Geometry check sheet. Reference: drawing and pictorial views, mm from the part's lowest x, y, z. A direction names the side the tool comes from. Coordinates: 2 decimals unless noted, no trailing zeros. Write each loop counter-clockwise with the first axis right and the second up, starting at its lowest first coordinate (ties: lowest second). Pieces come first, ordered by that corner, then holes.
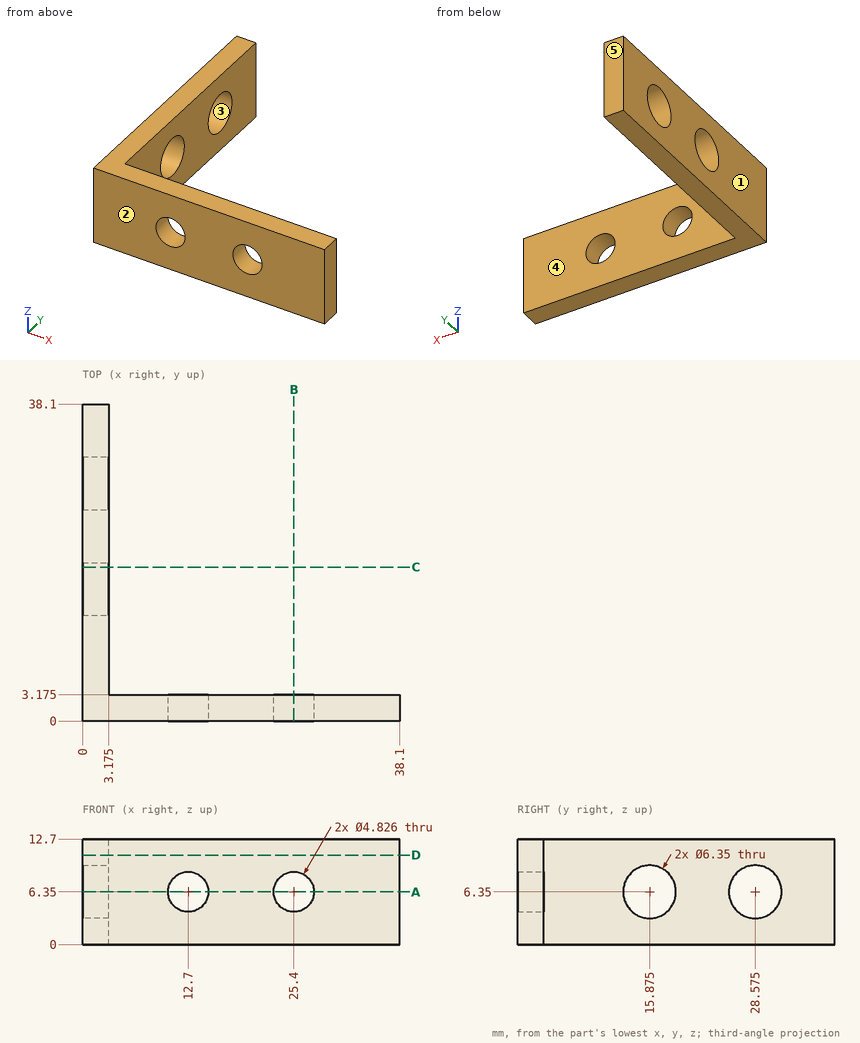
1. Sectioned sample at B-B, the plane x = 25.4. Record the boundary of the cut face in (y, z) (3 decimals).
2. Sectioned sample at D-D, the plane z = 10.75. Record the boundary of the cut face in (x, y) (3 decimals).
3. Material ranges on L1, parallel to X at y = 1.7, z = 6.35; L2, parallel to Y at x = 0.8, z = 6.35; L3, parallel to Y at x = 2, z = 4.25, recorded low to high.
4. Sectioned sample at C-C, the plane y = 18.5. Record the boundary of the cut face in (x, z) (3 decimals), and give its area (3 significant figures).
5. Draft check along Y on the marked faces 1, 2 and 3. Enter one of: pulls with the +Y half, pulls with the -Y half, needs draft (parallel to the pull), parting line crosses it, or undercut.
6. Gauge pin test, flat end, axial feed: P1, Ø1.5, axis at y = 20.5, z = 10, coming from the +X side (3 decimals). Record the tip position at first contact, or that the pin passes through.
7. Sectioned sample at A-A, the plane z = 6.35. Record the boundary of the cut face in (x, y) (3 decimals).
8. Tool access check on the marked faces 4 and 5. Record the directions out of +Z, -Z, +X, -X, +Y, -Y that give a thin tool (end or side, any length) a straight path to the whole face; none if there is none.
Outcome:
1. outline: (0, 0) - (3.175, 0) - (3.175, 3.937) - (0, 3.937) - close; (0, 8.763) - (3.175, 8.763) - (3.175, 12.7) - (0, 12.7) - close
2. outline: (0, 0) - (38.1, 0) - (38.1, 3.175) - (3.175, 3.175) - (3.175, 38.1) - (0, 38.1) - close
3. L1: x = 0 to 10.29, 15.11 to 22.99, 27.81 to 38.1
3. L2: y = 0 to 12.7, 19.05 to 25.4, 31.75 to 38.1
3. L3: y = 0 to 13.49, 18.26 to 26.19, 30.96 to 38.1
4. outline: (0, 0) - (3.175, 0) - (3.175, 4.564) - (0, 4.564) - close; (0, 8.136) - (3.175, 8.136) - (3.175, 12.7) - (0, 12.7) - close
4. area: 29.0 mm2
5. face 1: needs draft
5. face 2: pulls with the -Y half
5. face 3: undercut
6. P1: stops at x = 3.175
7. outline: (0, 0) - (10.287, 0) - (10.287, 3.175) - (3.175, 3.175) - (3.175, 12.7) - (0, 12.7) - close; (0, 19.05) - (3.175, 19.05) - (3.175, 25.4) - (0, 25.4) - close; (0, 31.75) - (3.175, 31.75) - (3.175, 38.1) - (0, 38.1) - close; (15.113, 0) - (22.987, 0) - (22.987, 3.175) - (15.113, 3.175) - close; (27.813, 0) - (38.1, 0) - (38.1, 3.175) - (27.813, 3.175) - close
8. face 4: +Z, -Z, +X, +Y
8. face 5: +Z, -Z, +X, -X, +Y
